The listing builds one solid part. Answer for the finished solid, in the listing's coordinates (mm). Face numbers are marked on the shaded views. A direction names the side the tool comes from. Round coordinates to 2 decimals unless told otherwise and drop trailing zeros. Write each loop counter-clockwise with the first axis right and the second up, starting at its lowest first coordinate (ties: lowest second). Pieces come first, ordered by that corner, then holes. Notation, with made-up numbers: M 17,-35.75 L 76,-35.75 A18 cw 76,-6.75 Z; hole C -21,12.25 d4. An arc over 180 degrees is marked long. Write each question's results on one line, items separated by ' | '.
from build123d import *

# Parameters (mm, degrees)
F0_R     = 12.7
F1_DEPTH = 25.4
F2_W     = 50.8
F2_H     = 127
F3_DEPTH = 50.8
F5_DEPTH = 127
F6_R     = 12.7
F7_DEPTH = 127
F8_W     = 63.5
F8_H     = 63.5
F9_DEPTH = 76.2


with BuildPart() as f1:
    # F0 (on Top) → F1 (new body)
    with BuildSketch(Plane.XY):
        with BuildLine():
            ThreePointArc((-38.1, -114.3), (0, -152.4), (38.1, -114.3))
            Line((38.1, -114.3), (38.1, 114.3))
            ThreePointArc((38.1, 114.3), (0, 152.4), (-38.1, 114.3))
            Line((-38.1, 114.3), (-38.1, -114.3))
        make_face()
        with Locations((0, -114.3)):
            Circle(F0_R, mode=Mode.SUBTRACT)
        with Locations((0, 114.3)):
            Circle(F0_R, mode=Mode.SUBTRACT)
    extrude(amount=F1_DEPTH)

    # F2 (on face) → F3 (join)
    with BuildSketch(Plane.XY.offset(25.4)):
        Rectangle(F2_W, F2_H)
    extrude(amount=F3_DEPTH)

    # F4 (on face) → F5 (join)
    with BuildSketch(Plane.XZ.offset(63.5)):
        with BuildLine():
            Line((-25.4, 76.2), (25.4, 76.2))
            ThreePointArc((25.4, 76.2), (0, 101.6), (-25.4, 76.2))
        make_face()
    extrude(amount=-F5_DEPTH)

    # F6 (on face) → F7 (cut)
    with BuildSketch(Plane.XZ.offset(63.5)):
        with Locations((0, 76.2)):
            Circle(F6_R)
    extrude(amount=-F7_DEPTH, mode=Mode.SUBTRACT)

    # F8 (on face) → F9 (cut)
    with BuildSketch(Plane.YZ.offset(25.4)):
        with BuildLine():
            Line((31.75, 76.2), (-31.75, 76.2))
            ThreePointArc((-31.75, 76.2), (0, 44.45), (31.75, 76.2))
        make_face()
        with Locations((0, 107.95)):
            Rectangle(F8_W, F8_H)
    extrude(amount=-F9_DEPTH, mode=Mode.SUBTRACT)


solid = f1.part
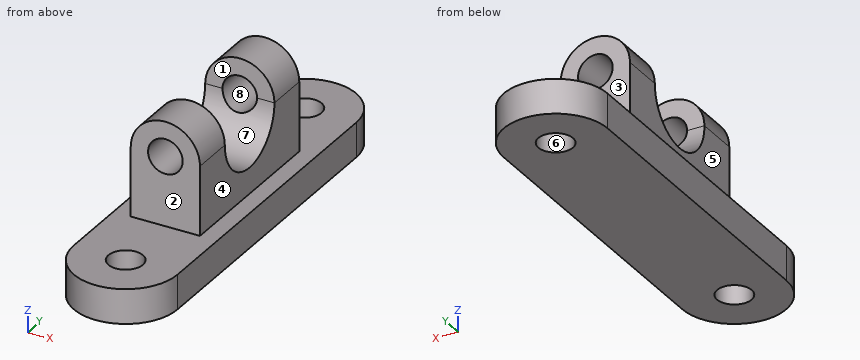
1) Section B-B (y = 110.5) is taken. Determine the outline of the cut face in (x, z), then the cut area to 3 significant figures.
Return value:
outline: M -38.1,0 L -12.12,0 L -12.12,25.4 L -38.1,25.4 Z; M 12.12,0 L 38.1,0 L 38.1,25.4 L 12.12,25.4 Z | area: 1,320 mm²
2) The mould has two halves that part along Z. Classify the marked faces 6, 7 and 8: +Z half, -Z half, draft (parallel to the pull), parting line (faces both ways), or undercut.
Return value:
face 6: draft | face 7: +Z half | face 8: undercut
3) Section D-D (z = 86) is taken. Determine the outline of the cut face in (x, y).
Return value:
outline: M -23.43,-63.5 L -8.08,-63.5 L -8.08,-31.75 L -23.43,-31.75 Z; M -23.43,31.75 L -8.08,31.75 L -8.08,63.5 L -23.43,63.5 Z; M 8.08,-63.5 L 23.43,-63.5 L 23.43,-31.75 L 8.08,-31.75 Z; M 8.08,31.75 L 23.43,31.75 L 23.43,63.5 L 8.08,63.5 Z
4) Each of these flat-tipped pins is pushed along its axis until it touches: pin 1 (7.5 mm diameter, centred on x = 5, z = 85.5, fed in from -Y); pin 2 (1 mm diameter, centred on x = -14.5, z = 57, fed in from +Y); pin 3 (4 mm diameter, centred on x = 22.5, z = 12, fed in from +Y); pin 4 (15 mm diameter, centred on x = 0, z = 76.2, fed in from -Y). Where does it stop, or does it pass through?
Return value:
pin 1: y = -63.5 | pin 2: y = 63.5 | pin 3: y = 146.41 | pin 4: through
5) Section C-C (z = 57) is taken. Determine the outline of the cut face in (x, y).
Return value:
outline: M -25.4,-63.5 L 25.4,-63.5 L 25.4,-25.29 L -25.4,-25.29 Z; M -25.4,25.29 L 25.4,25.29 L 25.4,63.5 L -25.4,63.5 Z
6) Section A-A (x = 0) is taken. Determine the outline of the cut face in (y, z), then the cut area to 3 significant figures.
Return value:
outline: M -152.4,0 L -127,0 L -127,25.4 L -152.4,25.4 Z; M -101.6,0 L 101.6,0 L 101.6,25.4 L 63.5,25.4 L 63.5,63.5 L 29.1,63.5 A31.75 cw -29.1,63.5 L -63.5,63.5 L -63.5,25.4 L -101.6,25.4 Z; M -63.5,88.9 L -31.75,88.9 L -31.75,101.6 L -63.5,101.6 Z; M 31.75,88.9 L 63.5,88.9 L 63.5,101.6 L 31.75,101.6 Z; M 127,0 L 152.4,0 L 152.4,25.4 L 127,25.4 Z | area: 11,300 mm²
7) Find the intervals of material crossed by line 1 (Y direction, x = 0, z = 20.5); line 2 (X direction, y = 52, z = 76.2); line 3 (Z direction, x = 10, y = 76), in increasing order.
Return value:
line 1: -152.4 to -127, -101.6 to 101.6, 127 to 152.4 | line 2: -25.4 to -12.7, 12.7 to 25.4 | line 3: 0 to 25.4
8) A tool of negligible diameter and unlimited length cuts with its end or side. For the marked faces 1, 2, 3, 4 and 5, from which of +Z, -Z, +X, -X, +Y, -Y can it reach the whole face along a straight path? Write none if from no direction.
Return value:
face 1: +Z, +X, -X | face 2: +Z, +X, -X, -Y | face 3: +Z, +X, -X, +Y | face 4: +Z, +X, +Y, -Y | face 5: +Z, -X, +Y, -Y
